Autodesk Inventor part; units mm, degrees
ref_plane "Work Plane1" through (0, 0, 5) normal (0, 0, 1) x (1, 0, 0)
ref_plane "Work Plane3" through (5, 0, 0) normal (1, 0, 0) x (0, 1, 0)
ref_plane "XZ Plane" through (0, 0, 0) normal (0, 1, 0) x (-1, 0, 0)
sketch "Sketch1" plane through (0, 0, 0) normal (0, 1, 0) x (-1, 0, 0)
  circle A0 centre (0, 0) radius 3.575
  circle A1 centre (0, 0) radius 5
  dimension "d0" = 7.15
  dimension "d1" = 10
extrude "Extrusion1" add sketch "Sketch1" along normal mid plane 40
ref_plane "Work Plane1" through (0, 0, 5) normal (0, 0, 1) x (1, 0, 0)
sketch "Sketch2" plane through (0, 0, 5) normal (0, 0, 1) x (1, 0, 0)
  circle A0 centre (0, 0) radius 3.575
  circle A1 centre (0, 0) radius 5
  line L0 (5, 20) -> (-5, 20)
  dimension "d4" = 7.15
  dimension "d5" = 10
  dimension "d22" = 0
extrude "Extrusion2" add sketch "Sketch2" along normal blind 15 and the other way blind 5
sketch "Sketch3" plane through (0, 0, 20) normal (0, 0, 1) x (1, 0, 0)
  circle A0 centre (0, 0) radius 3.575
extrude "Extrusion3" cut sketch "Sketch3" against normal up to surface
sketch "Sketch4" plane through (0, 20, 0) normal (0, 1, 0) x (1, 0, 0)
  circle A0 centre (0, 0) radius 3.615
  dimension "d13" = 7.23
extrude "Extrusion4" cut sketch "Sketch4" against normal through all
ref_plane "Work Plane3" through (5, 0, 0) normal (1, 0, 0) x (0, 1, 0)
sketch "Sketch6" plane through (5, 0, 0) normal (1, 0, 0) x (0, 1, 0)
  circle A0 centre (0, 0) radius 3.615
  circle A1 centre (0, 0) radius 5
  dimension "d23" = 7.23
  dimension "d24" = 10
extrude "Extrusion6" add sketch "Sketch6" along normal blind 15 and the other way blind 5
sketch "Sketch7" plane through (0, 0, 20) normal (0, 0, 1) x (1, 0, 0)
  circle A0 centre (0, 0) radius 3.615
  dimension "d33" = 7.23
extrude "Extrusion7" cut sketch "Sketch7" against normal up to surface
sketch "Sketch8" plane through (0, -20, 0) normal (0, -1, 0) x (1, 0, 0)
  circle A0 centre (0, 0) radius 3.615
extrude "Extrusion8" cut sketch "Sketch8" against normal through all
sketch "Sketch9" plane through (20, 0, 0) normal (1, 0, 0) x (0, 0, -1)
  line L0 (0, 0) -> (-2.5562, 2.5562)
  circle A0 centre (0, 0) radius 3.615
  dimension "d34" = 7.23
extrude "Extrusion9" cut sketch "Sketch9" against normal up to surface
sketch "Sketch5" plane through (0, 0, -5) normal (0, 0, 1) x (1, 0, 0)
  line L0 (5, 15) -> (-5, 15)
  line L1 (-5, -15) -> (5, -15)
  line L2 (2, 15) -> (-2, 15)
  line L3 (-2, 15) -> (-2, -15)
  line L4 (-2, -15) -> (2, -15)
  line L5 (2, -15) -> (2, 15)
  point P0 (0, 0)
  dimension "d16" = 4
  dimension "d17" = 2
properties part number "T-joint-UP"
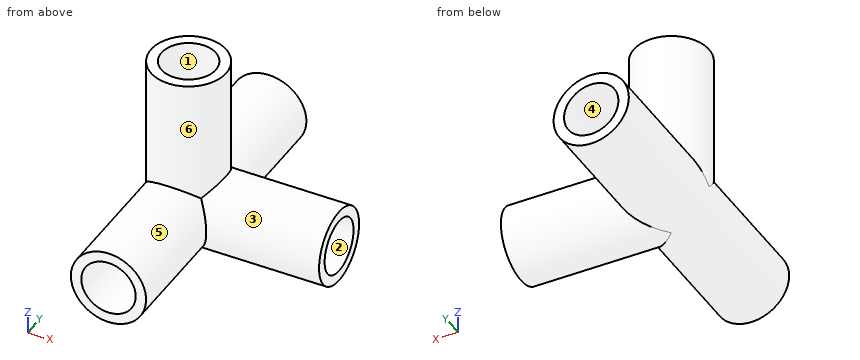
Geometry: final body of the model. Coordinates: model frame, mm. Face numbers are marked on the shaded views. A direction names the side the tool comes from. Give positions to 0.01 mm unless a question says otherwise; leave off trailing zeros. Write each loop counter-clockwise with the first axis right and the second up, starting at its lowest first coordinate (ties: lowest second). Pieces come first, ordered by that corner, then holes.
(1) First-contact query: P1, Ø8, axis at y = 9, z = 3.5, coming from the +X side; P2, Ø12, axis at x = 3.5, y = -13, coming from the +Z side; P3, Ø4.5, axis at y = 0, z = 0, coming from the +X side; P4, Ø8.5, axis at x = 0, z = 0, coming from the -Y side. Flat tips, straight axial feed; report the tip coordinate or a pass-through.
(2) Access query for the marked faces 5 and 6. Directions: +Z, -Z, +X, -X, +Y, -Y. A direction counts if a zero-diameter tool reaches every point of the face in a straight line with its end or side. Return the directions, or none.
(3) Mould query, pull axis Z, two halves, no side actions, for the marked faces 1, 2, 3 and 4. Classes: released by +Z, released by -Z, zero draft, split by the parting line, or undercut.
(4) Cut plane B-B, the plane x = 16.75. Return loops of the section in (y, z) (3 decimals), then the cut area to 3 significant figures.
(5) Cut plane A-A, the plane y = 0. Return loops of the section in (x, z) (3 decimals).
(6) Ray query, line 1 (X direction, y = 6, z = 0) (3 decimals); line 2 (Y direction, x = 3.25, z = 11). Return the intervals inside material, ascending.
Values follow:
1. P1: stops at x = 5
1. P2: stops at z = 5
1. P3: stops at x = -2.83
1. P4: stops at y = -20
2. face 5: none
2. face 6: +Z
3. face 1: zero draft
3. face 2: undercut
3. face 3: split by the parting line
3. face 4: undercut
4. outline: circle Ø10 at (0, 0); hole circle Ø7.23 at (0, 0)
4. area: 37.5 mm2
5. outline: (-5, 0) arc R5 ccw to (0, -5) - (20, -5) - (20, -3.615) - (0, -3.615) arc R3.615 cw to (-3.615, 0) - (-3.615, 20) - (-5, 20) - close; (3.615, 3.615) - (20, 3.615) - (20, 5) - (5, 5) - (5, 20) - (3.615, 20) - close
6. line 1: x = -5 to -3.615, 3.615 to 5
6. line 2: y = -3.8 to -1.58, 1.58 to 3.8
